Geometry check sheet. Reference: drawing and pictorial views, mm from the part's lowest x, y, z. A direction names the side the tool comes from. Give positions to 0.01 mm unless a question says otherwise; leave off trailing zeros. Order: outer loops, then holes, each group sorted by start corner. A loop starts at its lowest first (then second) coordinate and runs counter-clockwise, first axis right, second up.
Item 1: Sectioned sample at C-C on z = 0.65. Record the boundary of the cut face in (x, y).
Item 2: Sectioned sample at B-B on x = 16. Record the boundary of the cut face in (y, z).
Item 3: Gauge pin test, flat ends, axial feed: P1, Ø2, axis at y = 12, z = 1, coming from the -X side; P2, Ø0.5, axis at x = 20.5, z = 1.5, coming from the +Y side; P3, Ø3, axis at x = 9, y = 18, coming from the -Z side. Record the tip position at first contact, or that the pin passes through.
Item 4: Access from +Z, -Z, +X, -X, +Y, -Y to the whole of each face (thin tool, end or side, straight path). Record for the marked faces 1 and 2.
Item 5: Material ranges on line 1 along X through (y, z) = (8.5, 3.2); line 2 along Y through (x, z) = (31, 4.7); line 3 along Z through (x, y) = (7, 11), recorded low to high.
Item 6: Sectioned sample at A-A on y = 10. Record the boundary of the cut face in (x, z).
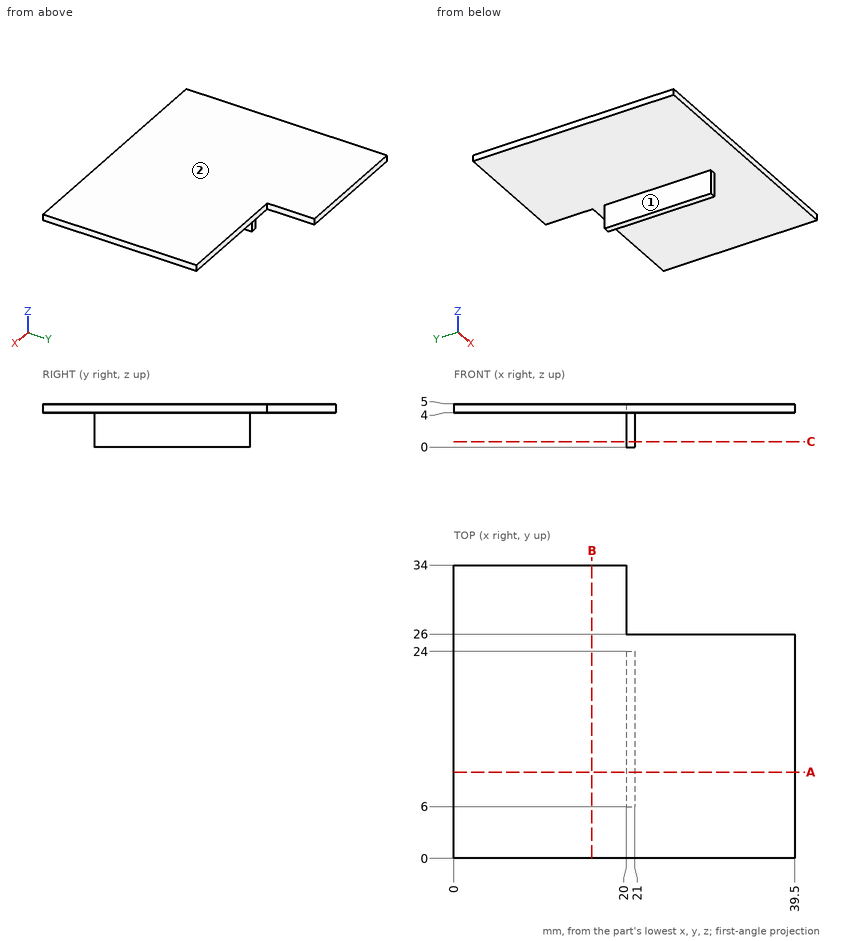
Report:
1. outline: (20, 6) - (21, 6) - (21, 24) - (20, 24) - close
2. outline: (0, 4) - (34, 4) - (34, 5) - (0, 5) - close
3. P1: stops at x = 20
3. P2: stops at y = 24
3. P3: stops at z = 4
4. face 1: -Z, -X, +Y, -Y
4. face 2: +Z, +X, -X, +Y, -Y
5. line 1: x = 20 to 21
5. line 2: y = 0 to 26
5. line 3: z = 4 to 5
6. outline: (0, 4) - (20, 4) - (20, 0) - (21, 0) - (21, 4) - (39.5, 4) - (39.5, 5) - (0, 5) - close
